Part model, mm, in its own coordinate system. A direction names the side the tool comes from. Give positions to 0.01 mm unless a question says otherwise; leave off trailing zeros. Order: outer loops, then holes, each group sorted by start corner. A loop starts at its lowest first (then second) coordinate and runs counter-clockwise, first axis right, second up. Notation, with made-up numbers: (-4.75, 81) - (3.25, 81) arc R13 ccw to (3.25, 93) - close; hole circle Ø9 at (57.5, 35.5). An arc over 180 degrees is marked (long way). One line per item, written item: value.
```python
from build123d import *

# Parameters (mm, degrees)
SKETCH_1_R        = 2.5
SKETCH_1_R_2      = 1.6
SKETCH_1_R_3      = 0.8
EXTRUDE_1_DEPTH   = 2
SKETCH_4_R        = 5
SKETCH_4_R_2      = 3
EXTRUDE_1_2_DEPTH = 3.6


with BuildPart() as part:
    # 草圖1 → Extrude 1 (new body)
    with BuildSketch(Plane(origin=(0, 0, 0), x_dir=(1, 0, 0), z_dir=(0, 1, 0))):
        with BuildLine():
            Line((0.636, 5.362415873), (22.823888889, 2.730859936))
            ThreePointArc((22.823888889, 2.730859936), (25.25, 0), (22.823888889, -2.730859936))
            Line((22.823888889, -2.730859936), (0.636, -5.362415873))
            ThreePointArc((0.636, -5.362415873), (-5.4, 0), (0.636, 5.362415873))
        make_face()
        Circle(SKETCH_1_R, mode=Mode.SUBTRACT)
        with Locations((8.8, 0)):
            Circle(SKETCH_1_R_2, mode=Mode.SUBTRACT)
        with Locations((14.2, 0)):
            Circle(SKETCH_1_R_3, mode=Mode.SUBTRACT)
        with Locations((18.3, 0)):
            Circle(SKETCH_1_R_3, mode=Mode.SUBTRACT)
        with Locations((22.5, 0)):
            Circle(SKETCH_1_R_3, mode=Mode.SUBTRACT)
    extrude(amount=EXTRUDE_1_DEPTH)

    # 草圖4 → Extrude 1 2 (add)
    with BuildSketch(Plane(origin=(0, 2, 0), x_dir=(1, 0, 0), z_dir=(0, 1, 0))):
        Circle(SKETCH_4_R)
        Circle(SKETCH_4_R_2, mode=Mode.SUBTRACT)
    extrude(amount=EXTRUDE_1_2_DEPTH)


solid = part.part
```
1) Cut at A-A, the plane z = 0. Give the number of separate pieces and of enclosed holes in the cut face, then the cut area to 3 significant figures.
Outcome:
separate pieces: 6
enclosed holes: 0
area: 49.7 mm^2
2) Mould opens along X. For faces 1 (the cylindrical face through (15, 1, 0)), 2 (the flat face through (11.575, 0.986, -4.065)), 3 (the cylindrical face through (-0.54, 0.99, 2.44)), 4 (the flat face through (14, 2, -1)) say: released by +X, released by -X, zero draft, split by the parting line, or undercut.
Outcome:
face 1: undercut
face 2: released by +X
face 3: undercut
face 4: zero draft
3) Cut at B-B, the plane x = 0. Give the cut face in (y, z).
Outcome:
outline: (0, -5.4) - (2, -5.4) - (2, -5) - (5.6, -5) - (5.6, -3) - (2, -3) - (2, -2.5) - (0, -2.5) - close; (0, 2.5) - (2, 2.5) - (2, 3) - (5.6, 3) - (5.6, 5) - (2, 5) - (2, 5.4) - (0, 5.4) - close
4) Pin check, flat tips, straight feed: pin 1 (1 mm diameter, centred on x = 18.3, z = 0, fed in from -Y); pin 2 (3 mm diameter, centred on x = 13, z = -1.5, fed in from +Y); pin 3 (1 mm diameter, centred on x = 9.5, y = 2, fed in from +Z); pin 4 (1.5 mm diameter, centred on y = 1, z = 2, fed in from +X). Stop position of each tip, or through.
Outcome:
pin 1: passes through
pin 2: stops at y = 2
pin 3: stops at z = 4.37
pin 4: stops at x = 24.95
5) Cut at C-C, the plane y = 1.55. Give the cut face in (x, z), then the cut area to 3 significant figures.
Outcome:
outline: (0.64, -5.36) - (22.82, -2.73) arc R2.75 ccw to (22.82, 2.73) - (0.64, 5.36) arc R5.4 ccw (long way) to start; hole circle Ø5 at (0, 0); hole circle Ø3.2 at (8.8, 0); hole circle Ø1.6 at (14.2, 0); hole circle Ø1.6 at (18.3, 0); hole circle Ø1.6 at (22.5, 0)
area: 209 mm^2
6) Drill centre lines: line 1 along X through (y, z) = (1.5, 0); line 2 along X through (y, z) = (0.85, 0.5); line 3 along Y through (x, z) = (16.5, -2.5). Where is each one in solid material? Low to high. Write a range as from..to.
Outcome:
line 1: x = -5.4..-2.5, 2.5..7.2, 10.4..13.4, 15..17.5, 19.1..21.7, 23.3..25.25
line 2: x = -5.38..-2.45, 2.45..7.28, 10.32..13.58, 14.82..17.68, 18.92..21.88, 23.12..25.2
line 3: y = 0..2
7) Which spindle directions (+Z, -Z, +X, -X, +Y, -Y) get a long thin tool onto all of the face, cutting with end or side? Do faces 5 (the cylindrical face through (-1.08, 3.77, 4.88)), 6 (the cylindrical face through (17.5, 1, 0)). Say none if no direction does.
Outcome:
face 5: +Y
face 6: +Y, -Y
8) Cut at D-D, the plane z = -1.25. Give the cut face in (x, y).
Outcome:
outline: (-5.25, 0) - (-2.17, 0) - (-2.17, 2) - (-2.73, 2) - (-2.73, 5.6) - (-4.84, 5.6) - (-4.84, 2) - (-5.25, 2) - close; (2.17, 0) - (7.8, 0) - (7.8, 2) - (4.84, 2) - (4.84, 5.6) - (2.73, 5.6) - (2.73, 2) - (2.17, 2) - close; (9.8, 0) - (24.95, 0) - (24.95, 2) - (9.8, 2) - close
